Design review of the part built by this model. Coordinates are the model's own, in mm. A direction names the side the tool comes from. Coordinates: 2 decimals unless noted, no trailing zeros. Loops run counter-clockwise (first coordinate to the right, second up) from the corner with the lowest first, then second, coordinate; pieces in that order, holes last. Notation, with made-up numbers: (47, 88) - (51, 88) arc R25 ccw to (51, 115) - close; hole circle Ø2 at (5, 84). An arc over 180 degrees is marked (long way). Answer in a Markdown table with one row per item. Add a question column.
(1) Clearance check with flat-ended pins moving along their axes: pin 1 (2 mm diameter, centred on x = 10.5, y = 1.5, fed in from -Z); pin 2 (1 mm diameter, centred on x = 11, y = 0.5, fed in from +Z). State where each tip first meets the part, or that it passes through.
(2) The part is to be moulded in two halves that separate along X. For faces 1 (the face through (7.861, -3.607, -0.017)), 2 (the face through (11.97, 0.07, -1.5)), 3 (the face through (9.7, 0.06, -1.4)), say which applies: released by +X, released by -X, zero draft, split by the parting line, or undercut.
(3) For faces 4 (the face through (9.194, 0, -2)), 5 (the face through (8.077, 1.007, -3.298)), list the 3-axis set-ups (+Z, -Z, +X, -X, +Y, -Y) from which the entire face can be reached by the end or side of a thin tool; tool diameter is ignored.
(4) We need section C-C, the plane x = 7.25. Write out the cut boundary in (y, z), plus the area to 3 significant figures.
(5) We need section A-A, the plane y = 0. Write out the cut boundary in (x, z).
(6) We need section D-D, the plane x = 8.25. Write out the cut boundary in (y, z), plus the area to 3 significant figures.
(7) To check wall thickness, follow L1, parallel to Y at x = 12, z = 0; L2, parallel to X at y = 0, z = 2.5; L3, parallel to Z at x = 7.75, y = -3. State the ranges of each line that lie inside material, in increasing order. Write a range as [from, to].
from build123d import *

# Parameters (mm, degrees)
F0_W     = 0.65359
F0_H     = 1.4
F0_W_2   = 3.5
F0_H_2   = 1.5
F3_DEPTH = 25


# Not quite as in the source:
# - ends of sketch curves that miss each other by under 0.0002 mm in the source are joined


with BuildPart() as f1:
    # F0 (on Front) → F1 (revolve)
    with BuildSketch(Plane.XZ):
        with BuildLine():
            ThreePointArc((9.366912, 1.4), (9.2669120175, 1.4267949091), (9.1937069394, 1.499999965))
            Line((9.193707, 1.499999965), (9.193707, 0))
            Line((9.193707, 0), (9.366912, 0))
            Line((9.366912, 0), (9.366912, 1.4))
        make_face()
        with Locations((9.693707, 0.7)):
            Rectangle(F0_W, F0_H)
        with BuildLine():
            ThreePointArc((10.1937070606, 1.499999965), (10.1205019825, 1.4267949091), (10.020502, 1.4))
            Line((10.020502, 1.4), (10.020502, 0))
            Line((10.020502, 0), (10.193707, 0))
            Line((10.193707, 0), (10.193707, 1.5))
        make_face()
        with Locations((11.943707, 0.75)):
            Rectangle(F0_W_2, F0_H_2)
        Polygon((14.193707, 1), (13.693707, 1.5), (13.693707, 0), (14.193707, 0), align=None)
        with BuildLine():
            Line((9.193707, 3.964102), (6.564298, 3.259553))
            ThreePointArc((6.5642979867, 3.2595530496), (6.2970304903, 3.0809709236), (6.193707, 2.77659))
            Line((6.193707, 2.77659), (6.193707, 0))
            Line((6.193707, 0), (9.193707, 0))
            Line((9.193707, 0), (9.193707, 1.499999965))
            Line((9.193707, 1.499999965), (9.193707, 3.964102))
        make_face()
    revolve(axis=Axis((10.368707, 0, 0), (-1, 0, 0)))

    # F2 (on face) → F3 (cut)
    with BuildSketch(Plane(origin=(6.193707, 0, 0), x_dir=(0, -1, 0), z_dir=(-1, 0, 0))):
        with BuildLine():
            ThreePointArc((3.8756311548, 0.8328191991), (2.8030435942, 2.8030432168), (0.8328197209, 3.8756310427))
            ThreePointArc((0.8328197209, 3.8756310427), (0.9707821759, 3.3957019848), (1.1674679485, 2.9367028921))
            ThreePointArc((1.1674679485, 2.9367028921), (1.3588439576, 2.5991932034), (1.5820188923, 2.2818124929))
            ThreePointArc((1.5820188923, 2.2818124929), (1.9633456176, 1.9633456176), (2.2818124929, 1.5820188923))
            ThreePointArc((2.2818124929, 1.5820188923), (2.599193614, 1.3588436976), (2.9367037599, 1.1674675107))
            ThreePointArc((2.9367037599, 1.1674675107), (3.3957025442, 0.9707819765), (3.8756311548, 0.8328191991))
        make_face()
        with BuildLine():
            ThreePointArc((-1.1674668381, 2.9367031109), (-0.9707811347, 3.3957021002), (-0.8328183948, 3.8756308663))
            ThreePointArc((-0.8328183948, 3.8756308663), (-2.8030431743, 2.8030436368), (-3.8756311107, 0.8328194045))
            ThreePointArc((-3.8756311107, 0.8328194045), (-3.3957018345, 0.970781873), (-2.9367033101, 1.167467233))
            ThreePointArc((-2.9367033101, 1.167467233), (-2.5991940372, 1.3588427967), (-2.281813665, 1.5820172017))
            ThreePointArc((-2.281813665, 1.5820172017), (-1.9633454104, 1.9633458247), (-1.5820167202, 2.2818139988))
            ThreePointArc((-1.5820167202, 2.2818139988), (-1.3588423817, 2.5991941131), (-1.1674668381, 2.9367031109))
        make_face()
        with BuildLine():
            ThreePointArc((2.2818124929, 1.5820188923), (1.9633456176, 1.9633456176), (1.5820188923, 2.2818124929))
            ThreePointArc((1.5820188923, 2.2818124929), (1.9101898753, 1.9101898753), (2.2818124929, 1.5820188923))
        make_face()
        with BuildLine():
            ThreePointArc((-2.281813665, 1.5820172017), (-1.9101891737, 1.9101895768), (-1.5820167202, 2.2818139988))
            ThreePointArc((-1.5820167202, 2.2818139988), (-1.9633454104, 1.9633458247), (-2.281813665, 1.5820172017))
        make_face()
        with BuildLine():
            ThreePointArc((-2.9367033101, -1.167467233), (-3.3957018345, -0.970781873), (-3.8756300769, -0.8328193482))
            ThreePointArc((-3.8756300769, -0.8328193482), (-2.8030431743, -2.8030436368), (-0.8328187651, -3.8756312481))
            ThreePointArc((-0.8328187651, -3.8756312481), (-0.9707811347, -3.3957021002), (-1.1674668381, -2.9367031109))
            ThreePointArc((-1.1674668381, -2.9367031109), (-1.3588423817, -2.5991941131), (-1.5820167202, -2.2818139988))
            ThreePointArc((-1.5820167202, -2.2818139988), (-1.9633454104, -1.9633458247), (-2.281813665, -1.5820172017))
            ThreePointArc((-2.281813665, -1.5820172017), (-2.5991940372, -1.3588427967), (-2.9367033101, -1.167467233))
        make_face()
        with BuildLine():
            ThreePointArc((0.8328197209, -3.8756310427), (2.8030435942, -2.8030432168), (3.8756311548, -0.8328191991))
            ThreePointArc((3.8756311548, -0.8328191991), (3.3957025442, -0.9707819765), (2.9367037599, -1.1674675107))
            ThreePointArc((2.9367037599, -1.1674675107), (2.599193614, -1.3588436976), (2.2818124929, -1.5820188923))
            ThreePointArc((2.2818124929, -1.5820188923), (1.9633456176, -1.9633456176), (1.5820188923, -2.2818124929))
            ThreePointArc((1.5820188923, -2.2818124929), (1.3588439576, -2.5991932034), (1.1674679485, -2.9367028921))
            ThreePointArc((1.1674679485, -2.9367028921), (0.9707821759, -3.3957019848), (0.8328197209, -3.8756310427))
        make_face()
        with BuildLine():
            ThreePointArc((1.5820188923, -2.2818124929), (1.9633456176, -1.9633456176), (2.2818124929, -1.5820188923))
            ThreePointArc((2.2818124929, -1.5820188923), (1.9101898753, -1.9101898753), (1.5820188923, -2.2818124929))
        make_face()
        with BuildLine():
            ThreePointArc((-1.5820167202, -2.2818139988), (-1.9101891737, -1.9101895768), (-2.281813665, -1.5820172017))
            ThreePointArc((-2.281813665, -1.5820172017), (-1.9633454104, -1.9633458247), (-1.5820167202, -2.2818139988))
        make_face()
    extrude(amount=-F3_DEPTH, mode=Mode.SUBTRACT)


solid = f1.part
Responses:
| question | item | result |
|---|---|---|
| 1 | pin 1 | stops at z = -1.41 |
| 1 | pin 2 | stops at z = 1.5 |
| 2 | face 1 | released by -X |
| 2 | face 2 | zero draft |
| 2 | face 3 | undercut |
| 3 | face 4 | +X |
| 3 | face 5 | -Z, +X, -X, +Y |
| 4 | outline | (-3.29, -1.01) arc R4 cw to (-2.94, -1.17) arc R4 cw to (-1.17, -2.94) arc R4 cw to (-1.01, -3.29) arc R3.44 ccw to (1.01, -3.29) arc R4 cw to (1.17, -2.94) arc R4 cw to (3.29, -1.01) arc R3.44 ccw to (3.29, 1.01) arc R4 cw to (2.94, 1.17) arc R4 cw to (1.01, 3.29) arc R3.44 ccw to (-1.01, 3.29) arc R4 cw to (-1.17, 2.94) arc R4 cw to (-2.94, 1.17) arc R4 cw to (-3.29, 1.01) arc R3.44 ccw to start |
| 4 | area | 30.8 mm2 |
| 5 | outline | (6.19, -2.78) arc R0.5 ccw to (6.56, -3.26) - (9.19, -3.96) - (9.19, -1.5) arc R0.2 cw to (9.37, -1.4) - (10.02, -1.4) arc R0.2 cw to (10.19, -1.5) - (13.69, -1.5) - (14.19, -1) - (14.19, 1) - (13.69, 1.5) - (10.19, 1.5) arc R0.2 cw to (10.02, 1.4) - (9.37, 1.4) arc R0.2 cw to (9.19, 1.5) - (9.19, 3.96) - (6.56, 3.26) arc R0.5 ccw to (6.19, 2.78) - close |
| 6 | outline | (-3.6, -0.9) arc R4 cw to (-2.94, -1.17) arc R4 cw to (-1.17, -2.94) arc R4 cw to (-0.9, -3.6) arc R3.71 ccw to (0.9, -3.6) arc R4 cw to (1.17, -2.94) arc R4 cw to (3.6, -0.9) arc R3.71 ccw to (3.6, 0.9) arc R4 cw to (2.94, 1.17) arc R4 cw to (0.9, 3.6) arc R3.71 ccw to (-0.9, 3.6) arc R4 cw to (-1.17, 2.94) arc R4 cw to (-2.94, 1.17) arc R4 cw to (-3.6, 0.9) arc R3.71 ccw to start |
| 6 | area | 32.9 mm2 |
| 7 | L1 | y = [-1.5, 1.5] |
| 7 | L2 | x = [6.19, 9.19] |
| 7 | L3 | z = [-1.14, 1.14] |
